Source: CAD feature listing. Evaluate the final solid. Frame: model axes, mm. Face numbers are marked on the shaded views. A direction names the side the tool comes from. Coordinates: 2 decimals unless noted, no trailing zeros. Loops run counter-clockwise (first coordinate to the right, second up) from the corner with the lowest first, then second, coordinate; pieces in that order, holes last. Notation, with made-up numbers: (-25.75, -32.5) - (18.25, -32.5) arc R28 cw to (18.25, 4.5) - close; hole circle Ø7 at (42, 67.25). An arc over 180 degrees is marked (long way). Use CSV: the item, a comma, the result in double quotes. Start each with the question number.
Autodesk Inventor part; units mm, degrees
ref_plane "YZ Plane" through (0, 0, 0) normal (1, 0, 0) x (0, 1, 0)
ref_plane "XZ Plane" through (0, 0, 0) normal (0, 1, 0) x (-1, 0, 0)
ref_plane "XY Plane" through (0, 0, 0) normal (0, 0, 1) x (1, 0, 0)
sketch "Sketch1" plane through (0, 0, 0) normal (0, 1, 0) x (-1, 0, 0)
  circle A0 centre (0, 0) radius 9
  circle A1 centre (5, 0) radius 6 construction
  line L0 (0, 0) -> (-3, -5.1962) construction
  line L1 (0, 0) -> (-3, 5.1962) construction
  line L2 (0, 0) -> (-6.6506, 0) construction
  circle A2 centre (-3, 5.1962) radius 1.5
  circle A3 centre (-3, -5.1962) radius 1.5
  circle A4 centre (5, 0) radius 2.75
  arc A5 (1.5, 1.3229) -> (1.5, -1.3229) centre (0, 0) ccw
  line L3 (1.5, 1.3229) -> (1.5, -1.3229)
  dimension "d0" = 18
  dimension "d1" = 5
  dimension "d2" = 12
  dimension "d3" = 60
  dimension "d4" = 6
  dimension "d5" = 3
  dimension "d6" = 3
  dimension "d7" = 5.5
  dimension "d9" = 4
  dimension "d10" = 1.5
extrude "Extrusion1" add sketch "Sketch1" against normal blind 3
properties part number "Carrier_top"
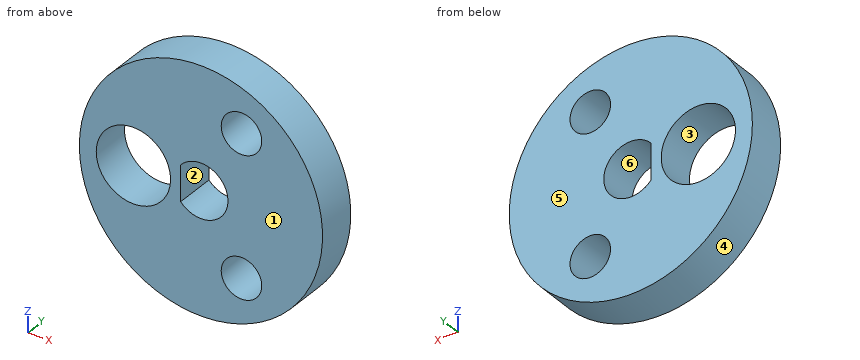
(1) Draft query along Z for the marked faces 3, 4, 5 and 6. Return one class per face: released by +Z, released by -Z, zero draft, split by the parting line, or undercut.
(2) Reachability of the marked faces 1 and 2 from +Z, -Z, +X, -X, +Y, -Y: full face, straight path, thin tool, end or side. Return the list, or none.
(3) Pin query (flat end, axial travel): pin 1 Ø2.5 at (x, z) = (3, -5.2) entering from -Y; pin 2 Ø1.5 at (y, z) = (-0.5, -6) entering from +X. Return the tip coordinate at first contact, or that it passes through.
(4) Section D-D on y = -0.45. Output: boundary loops of the cut face in (x, z).
(5) Section A-A on z = 0. Output: boundary loops of the cut face in (x, y).
(6) Section C-C on z = -2.25. Output: boundary loops of the cut face in (x, y).
(7) Section B-B on x = 0. Output: boundary loops of the cut face in (y, z), plus the area to 3 significant figures.
(8) Ray query, line 1 (Z direction, x = 0, y = -0.9); line 2 (Z direction, x = 2.75, y = -0.15); line 3 (Z direction, x = 3.5, y = -0.35). Return the intervals inside material, ascending. Write a range as [from, to].
Solution:
1,face 3,"undercut"
1,face 4,"split by the parting line"
1,face 5,"zero draft"
1,face 6,"undercut"
2,face 1,"+Z, -Z, +X, -X, -Y"
2,face 2,"+Y, -Y"
3,pin 1,"passes through"
3,pin 2,"stops at x = 7.31"
4,outline,"circle Ø18 at (0, 0); hole circle Ø5.5 at (-5, 0); hole (-1.5, -1.32) arc R2 ccw (long way) to (-1.5, 1.32) - close; hole circle Ø3 at (3, -5.2); hole circle Ø3 at (3, 5.2)"
5,outline,"(-9, -3) - (-7.75, -3) - (-7.75, 0) - (-9, 0) - close; (-2.25, -3) - (-1.5, -3) - (-1.5, 0) - (-2.25, 0) - close; (2, -3) - (9, -3) - (9, 0) - (2, 0) - close"
6,outline,"(-8.71, -3) - (-6.58, -3) - (-6.58, 0) - (-8.71, 0) - close; (-3.42, -3) - (8.71, -3) - (8.71, 0) - (-3.42, 0) - close"
7,outline,"(-3, -9) - (0, -9) - (0, -2) - (-3, -2) - close; (-3, 2) - (0, 2) - (0, 9) - (-3, 9) - close"
7,area,"42.0 mm²"
8,line 1,"z = [-9, -2], [2, 9]"
8,line 2,"z = [-8.57, -6.68], [-3.72, 3.72], [6.68, 8.57]"
8,line 3,"z = [-8.29, -6.61], [-3.78, 3.78], [6.61, 8.29]"
